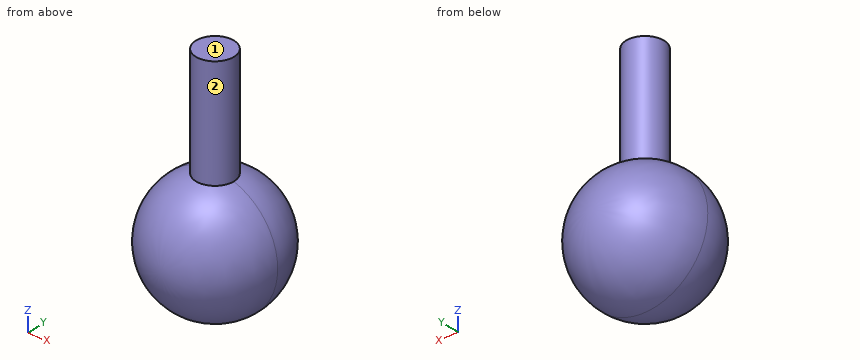
```python
from build123d import *

# Parameters (mm, degrees)
F0_R     = 50
F1_DEPTH = 50
F2_R     = 49.99999
F3_R     = 15
F4_DEPTH = 135


# Not quite as in the source:
# - a fillet or chamfer is up to 0.001 mm smaller than in the source, because OpenCascade refuses the exact size


with BuildPart() as f1:
    # F0 (on Front) → F1 (new body, symmetric)
    with BuildSketch(Plane.XZ):
        Circle(F0_R)
    extrude(amount=F1_DEPTH, both=True)

    # F2 (radius 50 in the source; OpenCascade refuses exactly that, so slightly less here)
    f2_edges = [f1.edges().sort_by_distance(p)[0] for p in [
        (-50, -50, 0),
        (-50, 50, 0),
    ]]
    fillet(f2_edges, radius=F2_R)

    # F3 (on Top) → F4 (join)
    with BuildSketch(Plane.XY):
        Circle(F3_R)
    extrude(amount=F4_DEPTH)


solid = f1.part
```
Input: part model. Units: mm. Frame: model coordinates. Face numbers are marked on the shaded views. Round coordinates to 2 decimals unless told otherwise and drop trailing zeros. One line per question, with ' | ' between items. Start each with the question number.
1) Pull-direction query (Y, two-part tool) for the marked faces 1 and 2; classes: +Y half, -Y half, draft (parallel to the pull), parting line (faces both ways), or undercut.
2) Ray query, probe 1 along X at (y, z) = (9, 117); probe 2 along Y at (x, z) = (-8.5, 19). Return the intervals inside material, ascending.
3) Contact query for flat-ended pins moving along their axis: P1, Ø8, axis at x = -23, z = -30.5, coming from the -Y side; P2, Ø6, axis at y = 16, z = 29.5, coming from the +X side; P3, Ø1.5, axis at y = -4.5, z = 11.5, coming from the +X side. Output: stop coordinate, or through.
Worked out:
1) face 1: draft | face 2: parting line
2) probe 1: x = -12 to 12 | probe 2: y = -45.46 to 45.46
3) P1: stops at y = -36.47 | P2: stops at x = 39.57 | P3: stops at x = 48.64
